```python
from build123d import *

# Parameters (mm, degrees)
SKETCH1_W           = 38.5
SKETCH1_H           = 23.75
BOSS_EXTRUDE1_DEPTH = 9.15
FILLET1_R           = 3
FILLET2_R           = 1.5


with BuildPart() as part:
    # Sketch1 → Boss-Extrude1 (new body)
    with BuildSketch(Plane(origin=(0, 0, 0), x_dir=(1, 0, 0), z_dir=(0, 1, 0))):
        Rectangle(SKETCH1_W, SKETCH1_H)
    extrude(amount=BOSS_EXTRUDE1_DEPTH)

    # Fillet1
    fillet1_edges = [part.edges().sort_by_distance(p)[0] for p in [
        (-19.25, 9.15, 0),
        (19.25, 9.15, 0),
        (-19.25, 0, 0),
        (19.25, 0, 0),
    ]]
    fillet(fillet1_edges, radius=FILLET1_R)

    # Fillet2
    fillet2_edges = [part.edges().sort_by_distance(p)[0] for p in [
        (-19.25, 4.575, 11.875),
        (-19.25, 4.575, -11.875),
        (0, 0, 11.875),
        (19.25, 4.575, 11.875),
        (0, 9.15, 11.875),
        (18.371320344, 8.271320344, 11.875),
        (18.371320344, 0.878679656, 11.875),
        (-18.371320344, 8.271320344, 11.875),
        (-18.371320344, 0.878679656, 11.875),
        (0, 0, -11.875),
        (0, 9.15, -11.875),
        (19.25, 4.575, -11.875),
        (18.371320344, 8.271320344, -11.875),
        (18.371320344, 0.878679656, -11.875),
        (-18.371320344, 8.271320344, -11.875),
        (-18.371320344, 0.878679656, -11.875),
    ]]
    fillet(fillet2_edges, radius=FILLET2_R)


solid = part.part
```
Build history of the part. All positions in model axes, mm. Give positions to 0.01 mm unless a question says otherwise; leave off trailing zeros. Order: outer loops, then holes, each group sorted by start corner. A loop starts at its lowest first (then second) coordinate and runs counter-clockwise, first axis right, second up. Notation, with made-up numbers: M 3.5,-8.5 L 39.5,-8.5 A25 cw 39.5,30.5 Z; hole C 42,-30.5 d1. An arc over 180 degrees is marked long. Write item = value, one per line. Start each with the question number.
(1) Probe L1, parallel to Z at x = -8, y = 7.75; L2, parallel to Y at x = -16.5, z = -5.5; L3, parallel to X at y = 7, z = 5.5. List the from-to ranges inside material, lowest first. Write a range as [from, to].
(2) Pin check, flat tip, straight feed: pin 1 Ø4 at (y, z) = (7.5, -7) entering from +X. Stop position of the tip, or through.
(3) Slice it at A-A on z = 1. Write the cut outline in (x, y).
Responses:
q1.L1 = [-11.87, 11.87]
q1.L2 = [0.01, 9.14]
q1.L3 = [-19.13, 19.13]
q2.pin_1 = 19.25
q3.outline = M -19.25,3 A3 ccw -16.25,0 L 16.25,0 A3 ccw 19.25,3 L 19.25,6.15 A3 ccw 16.25,9.15 L -16.25,9.15 A3 ccw -19.25,6.15 Z
